Work out the finished part from the listing and answer in its coordinate system (mm). A direction names the side the tool comes from. Coordinates: 2 decimals unless noted, no trailing zeros. Write each loop counter-clockwise with the first axis right and the second up, starting at its lowest first coordinate (ties: lowest second). Pieces come first, ordered by that corner, then holes. Notation, with made-up numbers: (-26, 82) - (-16, 82) arc R10 cw to (-16, 100) - close; hole circle Ø4 at (50, -11.5). An arc over 180 degrees is marked (long way). Use CSV: the item, a comma, the result in double quotes. Start each with the question number.
from build123d import *

# Parameters (mm, degrees)
SKETCH1_W           = 50.8
SKETCH1_H           = 19.05
BOSS_EXTRUDE1_DEPTH = 5.08
SKETCH2_W           = 10.16
SKETCH2_H           = 3.556
REVOLVE1_ANGLE      = 65


with BuildPart() as part:
    # Sketch1 → Boss-Extrude1 (new body)
    with BuildSketch(Plane(origin=(0, 0, 0), x_dir=(1, 0, 0), z_dir=(0, 1, 0))):
        with Locations((25.4, -9.525)):
            Rectangle(SKETCH1_W, SKETCH1_H)
    extrude(amount=BOSS_EXTRUDE1_DEPTH)

    # Sketch2 → Revolve1 (revolve)
    with BuildSketch(Plane(origin=(0, 5.08, 0), x_dir=(1, 0, 0), z_dir=(0, 1, 0))):
        with Locations((5.08, -17.272)):
            Rectangle(SKETCH2_W, SKETCH2_H)
        with Locations((45.72, -17.272)):
            Rectangle(SKETCH2_W, SKETCH2_H)
    revolve(axis=Axis((0, 5.08, 12.7), (-1, 0, 0)), revolution_arc=REVOLVE1_ANGLE)


solid = part.part
Item 1: A cutting plane is placed at B-B (x = 42). Determine the outline of the cut face in (y, z), then the cut area to 3 significant figures.
Item 2: A cutting plane is placed at D-D (z = 10). Determine the outline of the cut face in (x, y), then the cut area to 3 significant figures.
Item 3: Each of these flat-tipped pins is pushed along its axis until it touches: pin 1 (4 mm diameter, centred on x = 11.5, y = 8.5, fed in from +Z); pin 2 (1.5 mm diameter, centred on x = 35.5, z = 3.5, fed in from +Y). Where does it stop, or does it pass through?
Item 4: A cutting plane is placed at C-C (z = 14.5). Determine the outline of the cut face in (x, y).
Item 5: Determine the mould class of faces 3 (the face through (10.16, 7, 16)), 4 (the face through (45.79, 8.45, 18.08)), 5 (the face through (5.15, 6.56, 15.07)), 6 (the face through (45.79, 6.56, 15.07)) for opening direction Y: +Y half, -Y half, draft (parallel to the pull), parting line (faces both ways), or undercut.
Item 6: A cutting plane is placed at A-A (y = 7). Determine the outline of the cut face in (x, z), then the cut area to 3 significant figures.
Item 7: Which of the six approach directions +Z, -Z, +X, -X, +Y, -Y give full straight-line access (tool end or side, diameter ignored) to faces 1 (the face through (5.15, 8.45, 18.08)), 2 (the face through (40.64, 7, 16))?
Item 8: Straight lines are drawn through the part: probe 1 along Y at (x, z) = (30, 3); probe 2 along Z at (x, y) = (46, 6.5); probe 3 along Z at (x, y) = (6, 9.25). For each, find the intervals that lie inside material, in ascending order. Write a range as [from, to].
Calculated:
1,outline,"(0, 0) - (5.08, 0) - (5.08, 15.49) arc R2.79 cw to (7.61, 13.88) - (10.84, 15.38) arc R6.35 ccw to (5.08, 19.05) - (0, 19.05) - close"
1,area,"115 mm²"
2,outline,"(0, 0) - (50.8, 0) - (50.8, 5.08) - (0, 5.08) - close"
2,area,"258 mm²"
3,pin 1,"stops at z = 18.75"
3,pin 2,"stops at y = 5.08"
4,outline,"(0, 0) - (50.8, 0) - (50.8, 5.08) - (0, 5.08) - close; (0, 7.22) - (10.16, 7.22) - (10.16, 8.94) - (0, 8.94) - close; (40.64, 7.22) - (50.8, 7.22) - (50.8, 8.94) - (40.64, 8.94) - close"
5,face 3,"draft"
5,face 4,"+Y half"
5,face 5,"undercut"
5,face 6,"undercut"
6,outline,"(0, 14.73) - (10.16, 14.73) - (10.16, 18.75) - (0, 18.75) - close; (40.64, 14.73) - (50.8, 14.73) - (50.8, 18.75) - (40.64, 18.75) - close"
6,area,"81.7 mm²"
7,face 1,"+Z, +X, -X, +Y"
7,face 2,"+Z, -Z, +Y"
8,probe 1,"y = [0, 5.08]"
8,probe 2,"z = [15.11, 18.89]"
8,probe 3,"z = [14.64, 17.49]"
